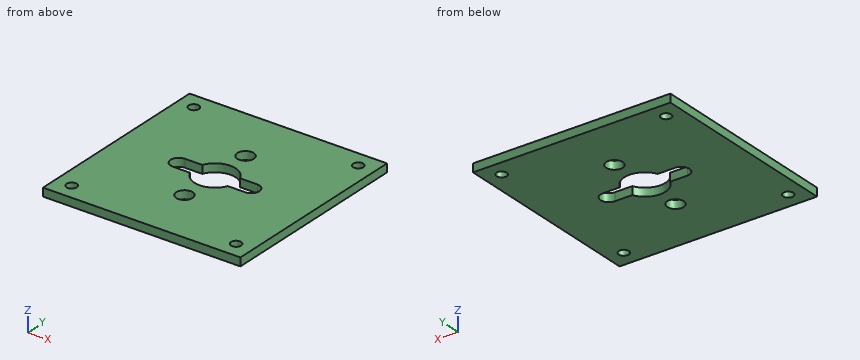
Autodesk Inventor part; units mm, degrees
ref_plane "YZ Plane" through (0, 0, 0) normal (1, 0, 0) x (0, 1, 0)
ref_plane "XZ Plane" through (0, 0, 0) normal (0, 1, 0) x (-1, 0, 0)
ref_plane "XY Plane" through (0, 0, 0) normal (0, 0, 1) x (1, 0, 0)
sketch "Sketch1" plane through (0, 0, 0) normal (0, 0, 1) x (1, 0, 0)
  line L0 (-38.1, 38.1) -> (38.1, 38.1)
  line L1 (38.1, 38.1) -> (38.1, -38.1)
  line L2 (38.1, -38.1) -> (-38.1, -38.1)
  line L3 (-38.1, -38.1) -> (-38.1, 38.1)
  circle A0 centre (0, 0) radius 7.9375
  line L4 (38.1, 38.1) -> (50.8, 38.1)
  line L5 (50.8, 38.1) -> (50.8, -38.1)
  line L6 (50.8, -38.1) -> (38.1, -38.1)
  line L7 (38.1, -38.1) -> (38.1, 38.1)
  line L8 (-38.1, 38.1) -> (-50.8, 38.1)
  line L9 (-50.8, 38.1) -> (-50.8, -38.1)
  line L10 (-50.8, -38.1) -> (-38.1, -38.1)
  line L11 (-38.1, -38.1) -> (-38.1, 38.1)
  arc A1 (-13.97, 3.175) -> (-13.97, -3.175) centre (-13.97, 0) ccw
  arc A2 (13.97, -3.175) -> (17.145, 0) centre (13.97, 0) ccw
  line L12 (-13.97, 3.175) -> (13.97, 3.175)
  arc A3 (17.145, 0) -> (13.97, 3.175) centre (13.97, 0) ccw
  line L13 (-13.97, -3.175) -> (13.97, -3.175)
  circle A4 centre (0, 15.875) radius 3.175
  circle A5 centre (0, -15.875) radius 3.175
  point P0 (-31.75, 31.75)
  point P1 (31.75, 31.75)
  point P2 (31.75, -31.75)
  point P3 (-31.75, -31.75)
  dimension "d0" = 76.2
  dimension "d1" = 76.2
  dimension "d2" = 38.1
  dimension "d3" = 38.1
  dimension "d4" = 15.875
  dimension "d5" = 6.35
  dimension "d6" = 6.35
  dimension "d7" = 6.35
  dimension "d8" = 6.35
  dimension "d36" = 12.7
  dimension "d37" = 12.7
  dimension "d42" = 6.35
  dimension "d43" = 27.94
  dimension "d44" = 3.175
  dimension "d45" = 13.97
  dimension "d46" = 6.35
  dimension "d47" = 6.35
  dimension "d48" = 15.875
  dimension "d49" = 31.75
extrude "Extrusion1" add sketch "Sketch1" against normal blind 3.175 contours L0 L1 L2 L3 | A0 L12 A3 A2 L13 | A0 L13 A1 L12 | A4 | A5
hole "Hole1" at (-31.75, 31.75, 0) at (31.75, 31.75, 0) at (31.75, -31.75, 0) at (-31.75, -31.75, 0) direction (0, 0, -1) diameter 3.9624 end through all
extrude "Extrusion3" cut sketch "Sketch1" against normal through all contours A0 L13 L12 | A0 L12 A3 A2 L13 | A0 L13 A1 L12 | A4 | A5
thread "Thread1"
thread "Thread2"
properties part number "Slide Plate BD Motor mount"
Work out the finished part from the listing and answer in its coordinate system (mm). Give positions to 0.01 mm unless a question says otherwise; leave off trailing zeros. Loops run counter-clockwise (first coordinate to the right, second up) from the corner with the lowest first, then second, coordinate; pieces in that order, holes last. Notation, with made-up numbers: (27.25, 74) -> (58.25, 74) arc R21 ccw to (58.25, 85) -> close; hole circle Ø11 at (71.25, 70.5). An arc over 180 degrees is marked (long way). Put each result on its own line as item: value. Start each with the question number.
Item 1: The part is cut by section B-B (x = -13). Give the vertices of the cut face in (y, z) (3 decimals).
Item 2: This flat-tipped pin is pushed along its axis until it touches: P1, Ø5, axis at x = 0, y = -15.875, coming from the +Z side. Where does it stop, or does it pass through?
Item 3: Find the intervals of material crossed by L1, parallel to X at y = -31.75, z = -1; L2, parallel to Y at x = 0, z = -2.35, in increasing order. Write a range as [from, to].
Item 4: The part is cut by section D-D (x = 0). State how many separate pieces and enclosed holes the cut face has, then the cut area to 3 significant figures.
Item 5: The part is cut by section C-C (y = 0). Give the vertices of the cut face in (x, z) (3 decimals), then the cut area to 3 significant figures.
Item 6: The part is cut by section A-A (y = -31.75). Give the vertices of the cut face in (x, z) (3 decimals), then the cut area to 3 significant figures.
Answers below:
1. outline: (-38.1, -3.175) -> (-3.175, -3.175) -> (-3.175, 0) -> (-38.1, 0) -> close; (3.175, -3.175) -> (38.1, -3.175) -> (38.1, 0) -> (3.175, 0) -> close
2. P1: through
3. L1: [-38.1, -33.73], [-29.77, 29.77], [33.73, 38.1]
3. L2: [-38.1, -19.05], [-12.7, -7.94], [7.94, 12.7], [19.05, 38.1]
4. separate pieces: 4
4. enclosed holes: 0
4. area: 151 mm2
5. outline: (-38.1, -3.175) -> (-17.145, -3.175) -> (-17.145, 0) -> (-38.1, 0) -> close; (17.145, -3.175) -> (38.1, -3.175) -> (38.1, 0) -> (17.145, 0) -> close
5. area: 133 mm2
6. outline: (-38.1, -3.175) -> (-33.731, -3.175) -> (-33.731, 0) -> (-38.1, 0) -> close; (-29.769, -3.175) -> (29.769, -3.175) -> (29.769, 0) -> (-29.769, 0) -> close; (33.731, -3.175) -> (38.1, -3.175) -> (38.1, 0) -> (33.731, 0) -> close
6. area: 217 mm2
